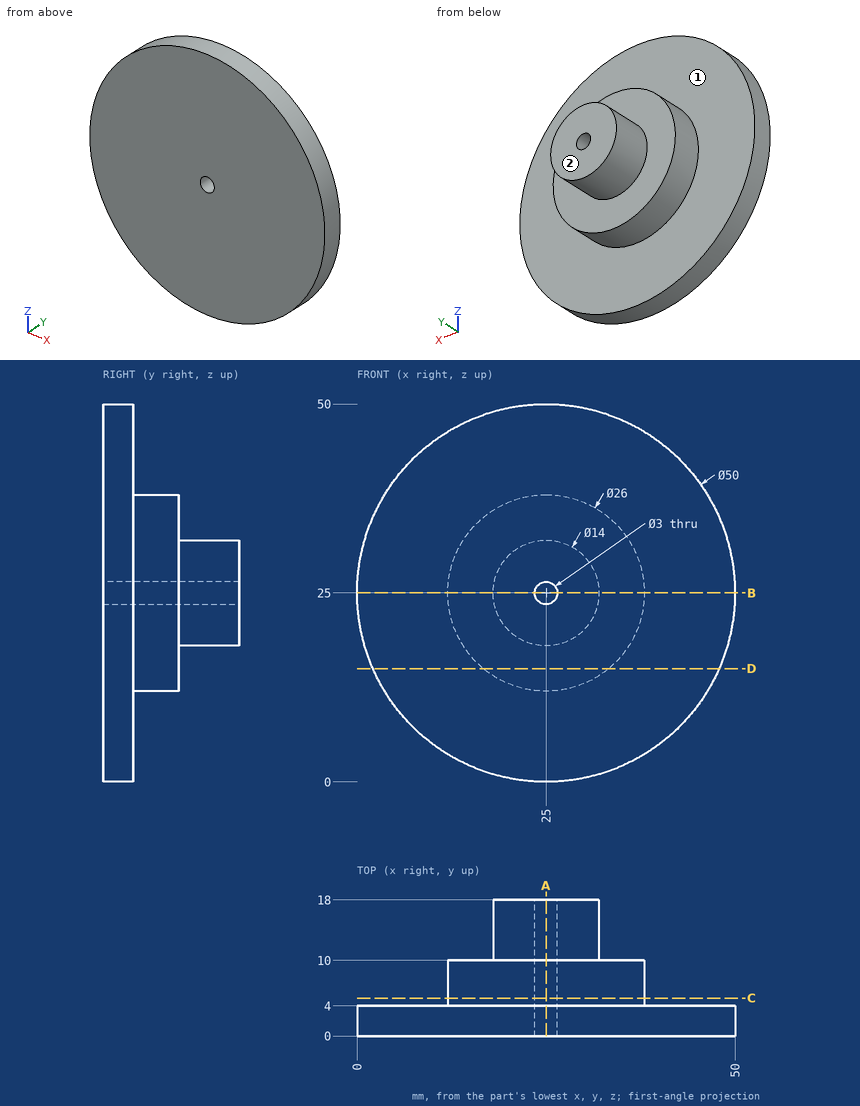
Job drawing, mm, ordinate dimensions from the low corner. One solid piece. A direction names the side the tool comes from. Give positions to 0.01 mm unless a question says otherwise; leave off trailing zeros. Loops run counter-clockwise (first coordinate to the right, second up) from the corner with the lowest first, then second, coordinate; pieces in that order, holes last. Notation, with made-up numbers: (-21.5, 45) -> (-15.5, 45) arc R23 cw to (-15.5, 75) -> close; hole circle Ø7 at (11, -24). An arc over 180 degrees is marked (long way). Use a Markdown table: item, result. Add a question column.
(1) Slice it at B-B on z = 25. List the corners of the cut face in (x, y).
(2) Slice it at C-C on y = 5. List the corners of the cut face in (x, z), and give its area (3 significant figures).
(3) Slice it at D-D on z = 15. List the corners of the cut face in (x, y).
(4) Drop flat-ended pins along their axis: pin 1 Ø3 at (y, z) = (9.5, 33.5) entering from +X; pin 2 Ø1 at (x, z) = (37, 35) entering from -Y; pin 3 Ø6 at (x, y) = (10.5, 2.5) entering from -Z; pin 4 Ø2 at (x, z) = (8, 25.5) entering from +Y. Give the stop position or say it passes through.
(5) Tool access for the marked faces 1 and 2: list every direction of +Z, -Z, +X, -X, +Y, -Y with a clear straight run to the whole face (end or side of a thin tool).
(6) Slice it at A-A on x = 25. List the corners of the cut face in (y, z).
(7) Wall check: line 1 along X through (y, z) = (6.25, 25); line 2 along X through (y, z) = (10.5, 25); line 3 along Y through (x, z) = (34.5, 10). Give the ranges that are in metal, low to high.
Filled sheet:
| question | item | result |
|---|---|---|
| 1 | outline | (0, 0) -> (23.5, 0) -> (23.5, 18) -> (18, 18) -> (18, 10) -> (12, 10) -> (12, 4) -> (0, 4) -> close; (26.5, 0) -> (50, 0) -> (50, 4) -> (38, 4) -> (38, 10) -> (32, 10) -> (32, 18) -> (26.5, 18) -> close |
| 2 | outline | circle Ø26 at (25, 25); hole circle Ø3 at (25, 25) |
| 2 | area | 524 mm2 |
| 3 | outline | (2.09, 0) -> (47.91, 0) -> (47.91, 4) -> (33.31, 4) -> (33.31, 10) -> (16.69, 10) -> (16.69, 4) -> (2.09, 4) -> close |
| 4 | pin 1 | x = 35.95 |
| 4 | pin 2 | y = 0 |
| 4 | pin 3 | z = 2.8 |
| 4 | pin 4 | y = 4 |
| 5 | face 1 | +Y |
| 5 | face 2 | +Z, -Z, +X, -X, +Y |
| 6 | outline | (0, 0) -> (4, 0) -> (4, 12) -> (10, 12) -> (10, 18) -> (18, 18) -> (18, 23.5) -> (0, 23.5) -> close; (0, 26.5) -> (18, 26.5) -> (18, 32) -> (10, 32) -> (10, 38) -> (4, 38) -> (4, 50) -> (0, 50) -> close |
| 7 | line 1 | 12 to 23.5, 26.5 to 38 |
| 7 | line 2 | 18 to 23.5, 26.5 to 32 |
| 7 | line 3 | 0 to 4 |
